Verification items for the finished model (mm, model axes). A direction names the side the tool comes from. Give positions to 0.01 mm unless a question says otherwise; leave off trailing zeros. Write each loop counter-clockwise with the first axis right and the second up, starting at its lowest first coordinate (ties: lowest second). Pieces come first, ordered by that corner, then holes. Notation, with made-up numbers: (-7, -17) -> (2, -17) arc R16 cw to (2, -7) -> close; hole circle Ø1 at (-23.75, 11.25). An arc over 180 degrees is marked (long way). Answer as CSV lines item,"result". Start each with the question number.
1) Sectioned sample at D-D on x = 640. Record the cut outline in (y, z), and give its area (3 significant figures).
2) Sectioned sample at A-A on z = -160. Record the cut outline in (x, y).
3) Tool access check on faces 1 (the flat face through (637, 177.8, -338)), 2 (the flat face through (787.4, -67, -338)), 3 (the flat face through (609.6, -455, 77)), 4 (the flat face through (-852, -177.8, -338)), 5 (the flat face through (482.6, 240, -338)). Record the directions out of +Z, -Z, +X, -X, +Y, -Y that give a thin tool (end or side, any length) a straight path to the whole face; none if there is none.
4) Mould release check, pull along X, two halves, no side actions. Record for faces 6 (the flat face through (850, -304.8, -338)), 7 (the cylindrical face through (882.264, -839.005, 77.267)), 8 (the flat face through (-787.4, 247, -338)): released by +X, released by -X, zero draft, split by the parting line, or undercut.
5) Sectioned sample at B-B on z = 22.5. Record the cut outline in (x, y).
6) Sectioned sample at C-C on y = -80.5. Record the cut outline in (x, z).
7) Material ranges on L1, parallel to Z at x = 388, y = 89; L2, parallel to Y at x = 552.5, z = -442; L3, parallel to X at y = -173, z = -404, recorded low to high.
8) Gauge pin test, flat ends, axial feed: pin 1 Ø4 at (x, z) = (681, -481) entering from -Y; pin 2 Ø3 at (y, z) = (99, -602) entering from -X. Record the tip position at first contact, or that the pin passes through.
```python
from build123d import *

# Parameters (mm, degrees)
F0_W     = 1828.8
F0_H     = 609.6
F1_DEPTH = 152.4
F2_W     = 127
F2_H     = 127
F2_H_2   = 116.919603
F3_DEPTH = 685.8
F5_DEPTH = 152.4


with BuildPart() as f1:
    # F0 (on Top) → F1 (new body)
    with BuildSketch(Plane.XY):
        Rectangle(F0_W, F0_H)
    extrude(amount=F1_DEPTH)

    # F2 (on face) → F3 (join)
    with BuildSketch(Plane(origin=(0, 0, 0), x_dir=(1, 0, 0), z_dir=(0, 0, -1))):
        with Locations((-850.9, 241.3)):
            Rectangle(F2_W, F2_H)
        with Locations((-850.9, -246.340198)):
            Rectangle(F2_W, F2_H_2)
        Polygon((787.4, -304.8), (914.4, -304.8), (914.4, 177.8), (914.4, 304.8), (787.4, 304.8), (787.4, -177.8), (482.6, -177.8), (482.6, -304.8), align=None)
    extrude(amount=F3_DEPTH)

    # F4 (on face) → F5 (join, through all)
    with BuildSketch(Plane.XY.offset(152.4)):
        with BuildLine():
            Line((914.4, -791.757951), (914.4, -304.8))
            Line((914.4, -304.8), (609.6, -304.8))
            Line((609.6, -304.8), (609.6, -609.6))
            Line((609.6, -609.6), (827.678976, -827.678976))
            ThreePointArc((827.678976, -827.678976), (883.040318, -838.691031), (914.4, -791.757951))
        make_face()
    extrude(amount=-F5_DEPTH)


solid = f1.part
```
Ans:
1,outline,"(-640, 0) -> (177.8, 0) -> (177.8, -685.8) -> (304.8, -685.8) -> (304.8, 152.4) -> (-640, 152.4) -> close"
1,area,"231,000 mm²"
2,outline,"(-914.4, -304.8) -> (-787.4, -304.8) -> (-787.4, -177.8) -> (-914.4, -177.8) -> close; (-914.4, 187.88) -> (-787.4, 187.88) -> (-787.4, 304.8) -> (-914.4, 304.8) -> close; (482.6, 177.8) -> (787.4, 177.8) -> (787.4, -304.8) -> (914.4, -304.8) -> (914.4, 304.8) -> (482.6, 304.8) -> close"
3,face 1,"-Z, -X, -Y"
3,face 2,"-Z, -Y"
3,face 3,"+Z, -Z, -X, -Y"
3,face 4,"-Z, -X"
3,face 5,"-Z, +Y, -Y"
4,face 6,"zero draft"
4,face 7,"split by the parting line"
4,face 8,"undercut"
5,outline,"(-914.4, -304.8) -> (609.6, -304.8) -> (609.6, -609.6) -> (827.68, -827.68) arc R50.8 ccw to (914.4, -791.76) -> (914.4, 304.8) -> (-914.4, 304.8) -> close"
6,outline,"(-914.4, 0) -> (787.4, 0) -> (787.4, -685.8) -> (914.4, -685.8) -> (914.4, 152.4) -> (-914.4, 152.4) -> close"
7,L1,"z = 0 to 152.4"
7,L2,"y = 177.8 to 304.8"
7,L3,"x = 787.4 to 914.4"
8,pin 1,"stops at y = 177.8"
8,pin 2,"stops at x = 787.4"
